```python
from build123d import *

# Parameters (mm, degrees)
SKETCH1_W               = 332.275
SKETCH1_H               = 146.5375
BOSS_EXTRUDE1_DEPTH     = 1.25
SKETCH2_W               = 332.275
SKETCH2_H               = 146.5375
SKETCH2_W_2             = 304.75
SKETCH2_H_2             = 119.0125
BOSS_EXTRUDE2_DEPTH     = 8
CHAMFER1_SIZE           = 1
M2_5_TAPPED_HOLE1_D     = 2.05
M2_5_TAPPED_HOLE1_DEPTH = 6.35
M2_5_TAPPED_HOLE1_TIP   = 0.615882135


with BuildPart() as part:
    # Sketch1 → Boss-Extrude1 (new, symmetric)
    with BuildSketch(Plane.XY):
        with Locations((161.924998435, 69.056249667)):
            Rectangle(SKETCH1_W, SKETCH1_H)
        with BuildLine():
            Line((313.799998435, 130.562499667), (292.299998435, 130.562499667))
            ThreePointArc((292.299998435, 130.562499667), (291.239338263, 131.001839495), (290.799998435, 132.062499667))
            Line((290.799998435, 132.062499667), (290.799998435, 132.562499667))
            ThreePointArc((290.799998435, 132.562499667), (285.799998435, 137.562499667), (280.799998435, 132.562499667))
            Line((280.799998435, 132.562499667), (280.799998435, 132.062499667))
            ThreePointArc((280.799998435, 132.062499667), (280.360658607, 131.001839495), (279.299998435, 130.562499667))
            Line((279.299998435, 130.562499667), (168.424998435, 130.562499667))
            ThreePointArc((168.424998435, 130.562499667), (167.364338263, 131.001839495), (166.924998435, 132.062499667))
            Line((166.924998435, 132.062499667), (166.924998435, 132.562499667))
            ThreePointArc((166.924998435, 132.562499667), (161.924998435, 137.562499667), (156.924998435, 132.562499667))
            Line((156.924998435, 132.562499667), (156.924998435, 132.062499667))
            ThreePointArc((156.924998435, 132.062499667), (156.485658607, 131.001839495), (155.424998435, 130.562499667))
            Line((155.424998435, 130.562499667), (44.549998435, 130.562499667))
            ThreePointArc((44.549998435, 130.562499667), (43.489338263, 131.001839495), (43.049998435, 132.062499667))
            Line((43.049998435, 132.062499667), (43.049998435, 132.562499667))
            ThreePointArc((43.049998435, 132.562499667), (38.049998435, 137.562499667), (33.049998435, 132.562499667))
            Line((33.049998435, 132.562499667), (33.049998435, 132.062499667))
            ThreePointArc((33.049998435, 132.062499667), (32.610658607, 131.001839495), (31.549998435, 130.562499667))
            Line((31.549998435, 130.562499667), (10.049998435, 130.562499667))
            ThreePointArc((10.049998435, 130.562499667), (8.282231482, 129.83026662), (7.549998435, 128.062499667))
            Line((7.549998435, 128.062499667), (7.549998435, 116.562499667))
            ThreePointArc((7.549998435, 116.562499667), (7.110658607, 115.501839495), (6.049998435, 115.062499667))
            Line((6.049998435, 115.062499667), (5.549998435, 115.062499667))
            ThreePointArc((5.549998435, 115.062499667), (0.549998435, 110.062499667), (5.549998435, 105.062499667))
            Line((5.549998435, 105.062499667), (6.049998435, 105.062499667))
            ThreePointArc((6.049998435, 105.062499667), (7.110658607, 104.623159839), (7.549998435, 103.562499667))
            Line((7.549998435, 103.562499667), (7.549998435, 34.549999667))
            ThreePointArc((7.549998435, 34.549999667), (7.110658607, 33.489339495), (6.049998435, 33.049999667))
            Line((6.049998435, 33.049999667), (5.549998435, 33.049999667))
            ThreePointArc((5.549998435, 33.049999667), (0.549998435, 28.049999667), (5.549998435, 23.049999667))
            Line((5.549998435, 23.049999667), (6.049998435, 23.049999667))
            ThreePointArc((6.049998435, 23.049999667), (7.110658607, 22.610659839), (7.549998435, 21.549999667))
            Line((7.549998435, 21.549999667), (7.549998435, 10.049999667))
            ThreePointArc((7.549998435, 10.049999667), (8.282231482, 8.282232714), (10.049998435, 7.549999667))
            Line((10.049998435, 7.549999667), (31.549998435, 7.549999667))
            ThreePointArc((31.549998435, 7.549999667), (32.610658607, 7.110659839), (33.049998435, 6.049999667))
            Line((33.049998435, 6.049999667), (33.049998435, 5.549999667))
            ThreePointArc((33.049998435, 5.549999667), (38.049998435, 0.549999667), (43.049998435, 5.549999667))
            Line((43.049998435, 5.549999667), (43.049998435, 6.049999667))
            ThreePointArc((43.049998435, 6.049999667), (43.489338263, 7.110659839), (44.549998435, 7.549999667))
            Line((44.549998435, 7.549999667), (155.424998435, 7.549999667))
            ThreePointArc((155.424998435, 7.549999667), (156.485658607, 7.110659839), (156.924998435, 6.049999667))
            Line((156.924998435, 6.049999667), (156.924998435, 5.549999667))
            ThreePointArc((156.924998435, 5.549999667), (161.924998435, 0.549999667), (166.924998435, 5.549999667))
            Line((166.924998435, 5.549999667), (166.924998435, 6.049999667))
            ThreePointArc((166.924998435, 6.049999667), (167.364338263, 7.110659839), (168.424998435, 7.549999667))
            Line((168.424998435, 7.549999667), (279.299998435, 7.549999667))
            ThreePointArc((279.299998435, 7.549999667), (280.360658607, 7.110659839), (280.799998435, 6.049999667))
            Line((280.799998435, 6.049999667), (280.799998435, 5.549999667))
            ThreePointArc((280.799998435, 5.549999667), (285.799998435, 0.549999667), (290.799998435, 5.549999667))
            Line((290.799998435, 5.549999667), (290.799998435, 6.049999667))
            ThreePointArc((290.799998435, 6.049999667), (291.239338263, 7.110659839), (292.299998435, 7.549999667))
            Line((292.299998435, 7.549999667), (313.799998435, 7.549999667))
            ThreePointArc((313.799998435, 7.549999667), (315.567765388, 8.282232714), (316.299998435, 10.049999667))
            Line((316.299998435, 10.049999667), (316.299998435, 21.549999667))
            ThreePointArc((316.299998435, 21.549999667), (316.739338263, 22.610659839), (317.799998435, 23.049999667))
            Line((317.799998435, 23.049999667), (318.299998435, 23.049999667))
            ThreePointArc((318.299998435, 23.049999667), (323.299998435, 28.049999667), (318.299998435, 33.049999667))
            Line((318.299998435, 33.049999667), (317.799998435, 33.049999667))
            ThreePointArc((317.799998435, 33.049999667), (316.739338263, 33.489339495), (316.299998435, 34.549999667))
            Line((316.299998435, 34.549999667), (316.299998435, 103.562499667))
            ThreePointArc((316.299998435, 103.562499667), (316.739338263, 104.623159839), (317.799998435, 105.062499667))
            Line((317.799998435, 105.062499667), (318.299998435, 105.062499667))
            ThreePointArc((318.299998435, 105.062499667), (323.299998435, 110.062499667), (318.299998435, 115.062499667))
            Line((318.299998435, 115.062499667), (317.799998435, 115.062499667))
            ThreePointArc((317.799998435, 115.062499667), (316.739338263, 115.501839495), (316.299998435, 116.562499667))
            Line((316.299998435, 116.562499667), (316.299998435, 128.062499667))
            ThreePointArc((316.299998435, 128.062499667), (315.567765388, 129.83026662), (313.799998435, 130.562499667))
        make_face(mode=Mode.SUBTRACT)
    extrude(amount=BOSS_EXTRUDE1_DEPTH, both=True)

    # Sketch2 → Boss-Extrude2 (add)
    with BuildSketch(Plane.XY.offset(1.25)):
        with Locations((161.924998435, 69.056249667)):
            Rectangle(SKETCH2_W, SKETCH2_H)
        with Locations((161.924998435, 69.056249667)):
            Rectangle(SKETCH2_W_2, SKETCH2_H_2, mode=Mode.SUBTRACT)
    extrude(amount=BOSS_EXTRUDE2_DEPTH)

    # Chamfer1
    chamfer1_edges = [part.edges().sort_by_distance(p)[0] for p in [
        (161.924998435, 9.549999667, 9.25),
        (9.549998435, 69.056249667, 9.25),
        (161.924998435, -4.212500333, 9.25),
        (328.062498435, 69.056249667, 9.25),
        (161.924998435, 142.324999667, 9.25),
        (-4.212501565, 69.056249667, 9.25),
        (161.924998435, 128.562499667, 9.25),
        (314.299998435, 69.056249667, 9.25),
    ]]
    chamfer(chamfer1_edges, length=CHAMFER1_SIZE)

    # M2.5 Tapped Hole1
    with Locations(Plane(origin=(0, 0, 1.25), x_dir=(-1, 0, 0), z_dir=(0, 0, -1))):
        with Locations((-285.799998435, 132.562499667), (-318.299998435, 110.062499667), (-318.299998435, 28.049999667), (-285.799998435, 5.549999667), (-161.924998435, 5.549999667), (-38.049998435, 5.549999667), (-5.549998435, 28.049999667), (-38.049998435, 132.562499667), (-5.549998435, 110.062499667), (-161.924998435, 132.562499667)):
            Hole(M2_5_TAPPED_HOLE1_D / 2, depth=M2_5_TAPPED_HOLE1_DEPTH)
            with Locations((0, 0, -(M2_5_TAPPED_HOLE1_DEPTH + M2_5_TAPPED_HOLE1_TIP / 2))):  # 118° drill point
                Cone(0, M2_5_TAPPED_HOLE1_D / 2, M2_5_TAPPED_HOLE1_TIP, mode=Mode.SUBTRACT)


solid = part.part
```
The model under review builds one solid part; all positions refer to its coordinate system, in mm. A direction names the side the tool comes from. Coordinates: 2 decimals unless noted, no trailing zeros. Write each loop counter-clockwise with the first axis right and the second up, starting at its lowest first coordinate (ties: lowest second). Pieces come first, ordered by that corner, then holes.
1) We need section A-A on y = 80. State the section outline as (x, z) points.
2) We need section C-C on z = 5.75. Count the separate pieces of the cut face and the enclosed holes in it, then the cut area to 3 significant figures.
3) Machinability: for faces 4 (the face through (160, -4.213, 3)), 5 (the face through (161, 130, 1.25)), 6 (the face through (160, 9.55, 5)), which of the approach directions +Z, -Z, +X, -X, +Y, -Y give a long, thin tool a straight path to every point of the face, cutting with its end or side? Answer none if there is none.
4) To check wall thickness, follow probe 1 along X at (y, z) = (69, -0.5); probe 2 along X at (y, z) = (82, 6.75). State the ranges of each line that lie inside material, in increasing order.
5) Clearance check with a flat-ended pin moving along its axis: pin 1 Ø2.5 at (x, y) = (285.8, 132.56) entering from -Z. State where the tip first meets the part, or that it passes through.
6) The part is to be moulded in two halves that separate along X. For faces 1 (the face through (149, 5, 9.25)), 2 (the face through (314.3, 68, 5)), 3 (the face through (-4.213, 68, 3)), say which applies: pulls with the +X half, pulls with the -X half, needs draft (parallel to the pull), parting line crosses it, or undercut.
Answer list:
1. outline: (-4.21, -1.25) - (7.55, -1.25) - (7.55, 1.25) - (9.55, 1.25) - (9.55, 8.25) - (8.55, 9.25) - (-3.21, 9.25) - (-4.21, 8.25) - close; (314.3, 1.25) - (316.3, 1.25) - (316.3, -1.25) - (328.06, -1.25) - (328.06, 8.25) - (327.06, 9.25) - (315.3, 9.25) - (314.3, 8.25) - close
2. separate pieces: 1
2. enclosed holes: 11
2. area: 12,400 mm2
3. face 4: +Z, -Z, +X, -X, -Y
3. face 5: -Z
3. face 6: +Z, -Z
4. probe 1: x = -4.21 to 7.55, 316.3 to 328.06
4. probe 2: x = -4.21 to 9.55, 314.3 to 328.06
5. pin 1: stops at z = 1.25
6. face 1: needs draft
6. face 2: undercut
6. face 3: pulls with the -X half
